Read the model definition and answer for the solid it produces. Units are mm, in the model's axes. A direction names the side the tool comes from. Give positions to 0.01 mm unless a question says otherwise; leave off trailing zeros. Order: outer loops, then holes, each group sorted by start corner. A loop starts at its lowest first (then second) coordinate and runs counter-clockwise, first axis right, second up. Notation, with made-up numbers: (-18.5, 0) -> (-9.5, 0) arc R38 ccw to (-9.5, 38) -> close; hole circle Ø8 at (-5, -25). An arc over 180 degrees is marked (long way). Use one line per item in the form item = value.
```python
from build123d import *

# Parameters (mm, degrees)
MODEL_R            = 0.5
EXTRUDE_1077_DEPTH = 8
FILLET_1_R         = 10
FILLET_2_R         = 1
HOLE_WIZARD_M2_D   = 1.6


with BuildPart() as part:
    # Model → Extrude 1077 (new body)
    with BuildSketch(Plane.XY):
        with BuildLine():
            Line((-32.875, 4), (-32.875, 11.86))
            Line((-32.875, 11.86), (-41.650081081, 11.86))
            ThreePointArc((-41.650081081, 11.86), (-50.430172197, 8.446970324), (-54.6, 0))
            Line((-54.6, 0), (0, 0))
            Line((0, 0), (60, 0))
            Line((60, 0), (60, 11.86))
            Line((60, 11.86), (47.375, 11.86))
            Line((47.375, 11.86), (47.375, 4))
            Line((47.375, 4), (43.375, 4))
            ThreePointArc((43.375, 4), (7.25, 6.986211556), (-28.875, 4))
            Line((-28.875, 4), (-32.875, 4))
        make_face()
        with Locations((-47.5, 2.93)):
            Circle(MODEL_R, mode=Mode.SUBTRACT)
        with Locations((55, 2.93)):
            Circle(MODEL_R, mode=Mode.SUBTRACT)
    extrude(amount=-EXTRUDE_1077_DEPTH)

    # Скругление1
    fillet_1_edges = [part.edges().sort_by_distance(p)[0] for p in [
        (60, 11.86, -4),
    ]]
    fillet(fillet_1_edges, radius=FILLET_1_R)

    # Скругление2
    fillet_2_edges = [part.edges().sort_by_distance(p)[0] for p in [
        (-54.6, 0, -4),
        (-32.875, 4, -4),
        (47.375, 4, -4),
        (60, 0, -4),
    ]]
    fillet(fillet_2_edges, radius=FILLET_2_R)

    # Крепление M2 (through all)
    with Locations(Plane.XY):
        with Locations((-47.5, 2.93), (55, 2.93)):
            Hole(HOLE_WIZARD_M2_D / 2)


solid = part.part
```
Item 1: The part is cut by section C-C on x = -12. Give the vertices of the cut face in (y, z).
Checks:
outline = (0, -8) -> (6.14, -8) -> (6.14, 0) -> (0, 0) -> close
Item 2: Given pin 1 Ø1.4 at (x, y) = (55, 2.93) entering from -Z; pin 2 Ø1.5 at (x, z) = (-13, -6) entering from +Y; pin 3 Ø3 at (x, z) = (-5, -6) entering from +Y; pin 4 Ø2 at (y, z) = (10, -6.5) entering from +X, each flat-ended and moving along its own axis, determine where each tip first touches the part or whether it passes through.
Checks:
pin_1 = through
pin_2 = 6.12
pin_3 = 6.72
pin_4 = 57
Item 3: Which of the six approach directions +Z, -Z, +X, -X, +Y, -Y give full straight-line access (tool end or side, diameter ignored) to faces 1 (the flat face through (45, 4, -4)), 2 (the flat face through (2, 0, -4))?
Checks:
face_1 = +Z, -Z, +Y
face_2 = +Z, -Z, +X, -X, -Y
Item 4: Determine the mould class of faces 3 (the cylindrical face through (-49.885, 8.919, -3.944)), 4 (the cylindrical face through (7.758, 6.986, -3.944)), 5 (the flat face through (-32.875, 8, -4)), 6 (the flat face through (-37, 11.86, -4)) for opening direction X: +X half, -X half, draft (parallel to the pull), parting line (faces both ways), or undercut.
Checks:
face_3 = -X half
face_4 = undercut
face_5 = undercut
face_6 = draft
Item 5: The part is cut by section A-A on z = -6. Give the vertices of the cut face in (x, y) (3 decimals).
Checks:
outline = (-54.442, 1.178) arc R1 ccw to (-53.458, 0) -> (59, 0) arc R1 ccw to (60, 1) -> (60, 1.86) arc R10 ccw to (50, 11.86) -> (47.375, 11.86) -> (47.375, 5) arc R1 cw to (46.375, 4) -> (43.375, 4) arc R220 ccw to (-28.875, 4) -> (-31.875, 4) arc R1 cw to (-32.875, 5) -> (-32.875, 11.86) -> (-41.65, 11.86) arc R13 ccw to start; hole circle Ø1.6 at (-47.5, 2.93); hole circle Ø1.6 at (55, 2.93)
Item 6: The part is cut by section B-B on x = 41. Give the vertices of the cut face in (y, z).
Checks:
outline = (0, -8) -> (4.38, -8) -> (4.38, 0) -> (0, 0) -> close
Item 7: Straight lines are drawn through the part: L1, parallel to X at y = 3.25, z = -3.5; L2, parallel to X at y = 2.25, z = -1; L3, parallel to Y at x = -47.5, z = -4.5. For each, find the intervals that lie inside material, in ascending order. Write a range as from..to.
Checks:
L1 = -53.89..-48.23, -46.77..54.27, 55.73..59.9
L2 = -54.2..-47.92, -47.08..54.58, 55.42..59.99
L3 = 0..2.13, 3.73..10.47
